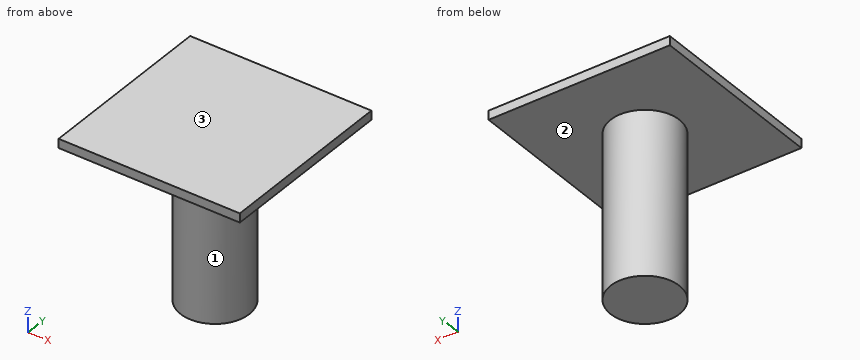
from build123d import *

# Parameters (mm, degrees)
F0_W     = 50
F0_H     = 50
F0_R     = 9.5
F1_DEPTH = 2.5
F2_DEPTH = 45


with BuildPart() as f1:
    # F0 (on Top) → F1 (new body)
    with BuildSketch(Plane.XY):
        with Locations((25, 31.013934)):
            Rectangle(F0_W, F0_H)
        with Locations((25, 31.013934)):
            Circle(F0_R, mode=Mode.SUBTRACT)
        with Locations((25, 31.013934)):
            Circle(F0_R)
    extrude(amount=F1_DEPTH)

    # F0 (on Top) → F2 (join)
    with BuildSketch(Plane.XY):
        with Locations((25, 31.013934)):
            Circle(F0_R)
    extrude(amount=-F2_DEPTH)


solid = f1.part
Design review of the part built by this model. Coordinates are the model's own, in mm. Face numbers are marked on the shaded views. Give positions to 0.01 mm unless a question says otherwise; leave off trailing zeros. Loops run counter-clockwise (first coordinate to the right, second up) from the corner with the lowest first, then second, coordinate; pieces in that order, holes last. Notation, with made-up numbers: M 83.25,60 L 123.25,60 A28 cw 123.25,92 Z; hole C -7.5,57.5 d5. An arc over 180 degrees is marked long. Write item = value, one per line.
Q1. We need section C-C (y = 15). Give the boundary of the cut face in (x, z).
Output values:
outline = M 0,0 L 50,0 L 50,2.5 L 0,2.5 Z
Q2. We need section D-D (z = -33.5). Give the boundary of the cut face in (x, y).
Output values:
outline = C 25,31.01 d19
Q3. We need section B-B (y = 38). Give the boundary of the cut face in (x, z), plus the area to 3 significant figures.
Output values:
outline = M 0,0 L 18.56,0 L 18.56,-45 L 31.44,-45 L 31.44,0 L 50,0 L 50,2.5 L 0,2.5 Z
area = 704 mm^2
Q4. Draft analysis for pull direction Z (two halves, no side actions). For the marked faces 1, 2 and 3, state which applies: +Z half, -Z half, draft (parallel to the pull), parting line (faces both ways), or undercut.
Output values:
face_1 = draft
face_2 = -Z half
face_3 = +Z half
Q5. We need section A-A (x = 25). Give the boundary of the cut face in (y, z).
Output values:
outline = M 6.01,0 L 21.51,0 L 21.51,-45 L 40.51,-45 L 40.51,0 L 56.01,0 L 56.01,2.5 L 6.01,2.5 Z
Q6. Insertion check: pin 1 (4 mm diameter, centred on x = 21.5, y = 17.5, fed in from -Z); pin 2 (12 mm diameter, centred on y = 43, z = -22, fed in from -X); pin 3 (10 mm diameter, centred on y = 36.5, z = -5.5, fed in from -X). Each pin has a flat end and moves straight along its axis. Give the tip position at first contact, or say it passes through.
Output values:
pin_1 = 0
pin_2 = 17.62
pin_3 = 15.51
Q7. To check wall thickness, follow line 1 (Z direction, x = 13.5, y = 38.5); line 2 (X direction, y = 28, z = -21); line 3 (X direction, y = 25, z = -32). State the ranges of each line that lie inside material, in increasing order. Write a range as [from, to].
Output values:
line_1 = [0, 2.5]
line_2 = [15.99, 34.01]
line_3 = [17.65, 32.35]
